```python
from build123d import *

# Parameters (mm, degrees)
BOSS_EXTRUDE1_DEPTH       = 6.35
SKETCH5_R                 = 6.35
CUT_EXTRUDE1_DEPTH        = 202.906036314
SKETCH6_W                 = 95.25
SKETCH6_H                 = 38.1
SKETCH6_W_2               = 107.95
CUT_EXTRUDE2_DEPTH        = 10.16
SKETCH7_W                 = 25.4
SKETCH7_H                 = 88.9
CUT_EXTRUDE3_DEPTH        = 3.175
M5X0_8_TAPPED_HOLE1_D     = 4.2
M5X0_8_TAPPED_HOLE1_DEPTH = 13.97
M5X0_8_TAPPED_HOLE1_TIP   = 1.2618073


with BuildPart() as part:
    # Sketch2 → Boss-Extrude1 (new body)
    with BuildSketch(Plane.XY):
        Polygon((184.15, -82.55), (184.15, 82.55), (0, 82.55), (0, -6.35), (31.75, -6.35), (31.75, -82.55), align=None)
    extrude(amount=BOSS_EXTRUDE1_DEPTH)

    # Sketch5 → Cut-Extrude1 (cut, through all)
    with BuildSketch(Plane.XY.offset(6.35)):
        with Locations((-158.75, 57.15)):
            Circle(SKETCH5_R)
        with Locations((-158.75, -57.15)):
            Circle(SKETCH5_R)
        with Locations((158.75, 57.15)):
            Circle(SKETCH5_R)
        with Locations((158.75, -57.15)):
            Circle(SKETCH5_R)
    extrude(amount=-CUT_EXTRUDE1_DEPTH, mode=Mode.SUBTRACT)

    # Sketch6 → Cut-Extrude2 (cut)
    with BuildSketch(Plane.XY.offset(6.35)):
        with Locations((98.425, -38.1)):
            Rectangle(SKETCH6_W, SKETCH6_H)
        with Locations((92.075, 38.1)):
            Rectangle(SKETCH6_W_2, SKETCH6_H)
    extrude(amount=-CUT_EXTRUDE2_DEPTH, mode=Mode.SUBTRACT)

    # Sketch7 → Cut-Extrude3 (cut)
    with BuildSketch(Plane(origin=(0, 0, 0), x_dir=(-1, 0, 0), z_dir=(0, 0, -1))):
        with Locations((-12.7, 38.1)):
            Rectangle(SKETCH7_W, SKETCH7_H)
    extrude(amount=-CUT_EXTRUDE3_DEPTH, mode=Mode.SUBTRACT)

    # M5x0.8 Tapped Hole1
    with Locations(Plane(origin=(0, 0, 3.175), x_dir=(-1, 0, 0), z_dir=(0, 0, -1))):
        with Locations((-12.7, 38.1), (-12.7, 63.5), (-12.7, 12.7), (-2.670853236, 86.574215023)):
            Hole(M5X0_8_TAPPED_HOLE1_D / 2, depth=M5X0_8_TAPPED_HOLE1_DEPTH)
            with Locations((0, 0, -(M5X0_8_TAPPED_HOLE1_DEPTH + M5X0_8_TAPPED_HOLE1_TIP / 2))):  # 118° drill point
                Cone(0, M5X0_8_TAPPED_HOLE1_D / 2, M5X0_8_TAPPED_HOLE1_TIP, mode=Mode.SUBTRACT)


solid = part.part
```
Check sheet for the modelled part. Datum: model origin and axes. Units: mm. A direction names the side the tool comes from. Coordinates: 2 decimals unless noted, no trailing zeros. Loops run counter-clockwise (first coordinate to the right, second up) from the corner with the lowest first, then second, coordinate; pieces in that order, holes last.
1) Release check for a two-part mould opening along Y. For faces 4 (the face through (104, 1, 0)), 5 (the face through (98, -19.05, 3)), 6 (the face through (19, -6.35, 5)) record: released by +Y, released by -Y, zero draft, split by the parting line, or undercut.
2) Sectioned sample at C-C (x = 12.7). Record the boundary of the cut face in (y, z) (3 decimals).
3) Material ranges on probe 1 along Y at (x, z) = (12.7, 4.5); probe 2 along Y at (x, z) = (145.5, 2); probe 3 along X at (y, z) = (57, 5.5), recorded low to high.
4) Sectioned sample at D-D (x = 43). Record the boundary of the cut face in (y, z), and give its area (3 significant figures).
5) Sectioned sample at A-A (x = 126). Record the boundary of the cut face in (y, z), and give its area (3 significant figures).
6) Gauge pin test, flat ends, axial feed: pin 1 (3 mm diameter, centred on x = 95, y = 19, fed in from -Z); pin 2 (3.5 mm diameter, centred on y = 48, z = 1, fed in from -X); pin 3 (12 mm diameter, centred on x = 124.5, y = 47, fed in from +Z); pin 4 (1.9 mm diameter, centred on y = -37.5, z = 3, fed in from -X). Record the tip position at first contact, or that the pin passes through.
7) Sectioned sample at B-B (y = -37). Record the boundary of the cut face in (x, z), and give its area (3 significant figures).
8) Access from +Z, -Z, +X, -X, +Y, -Y to the whole of each face (thin tool, end or side, straight path). Record for faces 1 (the face through (91, 1, 6.35)), 2 (the face through (146.05, -38, 3)), 3 (the face through (10, 39, 3.175)).
Check sheet entries:
1. face 4: zero draft
1. face 5: undercut
1. face 6: released by -Y
2. outline: (-6.35, 3.175) - (10.6, 3.175) - (10.6, 6.35) - (-6.35, 6.35) - close; (14.8, 3.175) - (36, 3.175) - (36, 6.35) - (14.8, 6.35) - close; (40.2, 3.175) - (61.4, 3.175) - (61.4, 6.35) - (40.2, 6.35) - close; (65.6, 3.175) - (82.55, 3.175) - (82.55, 6.35) - (65.6, 6.35) - close
3. probe 1: y = -6.35 to 10.6, 14.8 to 36, 40.2 to 61.4, 65.6 to 82.55
3. probe 2: y = -82.55 to -57.15, -19.05 to 19.05, 57.15 to 82.55
3. probe 3: x = 0 to 38.1, 146.05 to 152.4, 165.1 to 184.15
4. outline: (-82.55, 0) - (19.05, 0) - (19.05, 6.35) - (-82.55, 6.35) - close; (57.15, 0) - (82.55, 0) - (82.55, 6.35) - (57.15, 6.35) - close
4. area: 806 mm2
5. outline: (-82.55, 0) - (-57.15, 0) - (-57.15, 6.35) - (-82.55, 6.35) - close; (-19.05, 0) - (19.05, 0) - (19.05, 6.35) - (-19.05, 6.35) - close; (57.15, 0) - (82.55, 0) - (82.55, 6.35) - (57.15, 6.35) - close
5. area: 565 mm2
6. pin 1: stops at z = 0
6. pin 2: stops at x = 25.4
6. pin 3: passes through
6. pin 4: stops at x = 31.75
7. outline: (31.75, 0) - (50.8, 0) - (50.8, 6.35) - (31.75, 6.35) - close; (146.05, 0) - (184.15, 0) - (184.15, 6.35) - (146.05, 6.35) - close
7. area: 363 mm2
8. face 1: +Z, +X, -X, +Y, -Y
8. face 2: +Z, -Z
8. face 3: -Z, -X, +Y, -Y
